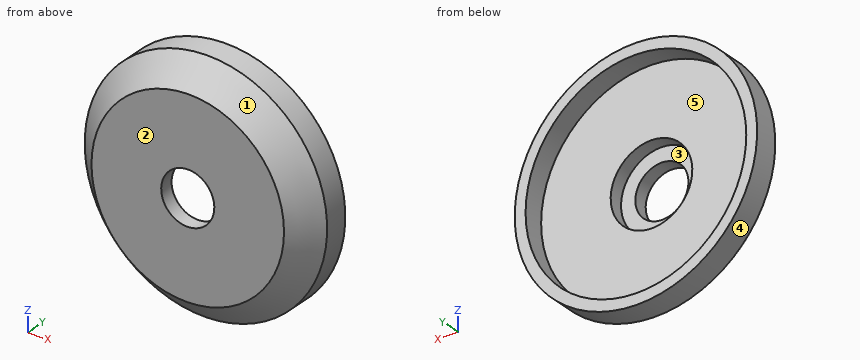
```python
from build123d import *

# Parameters (mm, degrees)
SKETCH1_R           = 34
BOSS_EXTRUDE1_DEPTH = 14
SKETCH2_R           = 30.95
CUT_EXTRUDE1_DEPTH  = 6
SKETCH3_R           = 11.45
CUT_EXTRUDE2_DEPTH  = 4
SKETCH4_R           = 7.45
CUT_EXTRUDE3_DEPTH  = 4
CHAMFER1_SIZE       = 7


with BuildPart() as part:
    # Sketch1 → Boss-Extrude1 (new body)
    with BuildSketch(Plane(origin=(0, 0, 0), x_dir=(1, 0, 0), z_dir=(0, 1, 0))):
        with Locations(Location((0, 0, 0), (0, 0, 270))):
            Circle(SKETCH1_R)
    extrude(amount=BOSS_EXTRUDE1_DEPTH)

    # Sketch2 → Cut-Extrude1 (cut)
    with BuildSketch(Plane(origin=(0, 14, 0), x_dir=(1, 0, 0), z_dir=(0, 1, 0))):
        with Locations(Location((0, 0, 0), (0, 0, 270))):
            Circle(SKETCH2_R)
    extrude(amount=-CUT_EXTRUDE1_DEPTH, mode=Mode.SUBTRACT)

    # Sketch3 → Cut-Extrude2 (cut)
    with BuildSketch(Plane(origin=(0, 8, 0), x_dir=(1, 0, 0), z_dir=(0, 1, 0))):
        with Locations(Location((0, 0, 0), (0, 0, 270))):
            Circle(SKETCH3_R)
    extrude(amount=-CUT_EXTRUDE2_DEPTH, mode=Mode.SUBTRACT)

    # Sketch4 → Cut-Extrude3 (cut)
    with BuildSketch(Plane(origin=(0, 4, 0), x_dir=(1, 0, 0), z_dir=(0, 1, 0))):
        with Locations(Location((0, 0, 0), (0, 0, 270))):
            Circle(SKETCH4_R)
    extrude(amount=-CUT_EXTRUDE3_DEPTH, mode=Mode.SUBTRACT)

    # Chamfer1
    chamfer1_edges = [part.edges().sort_by_distance(p)[0] for p in [
        (0, 0, -34),
    ]]
    chamfer(chamfer1_edges, length=CHAMFER1_SIZE)


solid = part.part
```
Part model, mm, in its own coordinate system. Face numbers are marked on the shaded views. A direction names the side the tool comes from. Round coordinates to 2 decimals unless told otherwise and drop trailing zeros. Order: outer loops, then holes, each group sorted by start corner. A loop starts at its lowest first (then second) coordinate and runs counter-clockwise, first axis right, second up. Notation, with made-up numbers: M -11.75,43 L 42.25,43 A22 ccw 42.25,68 Z; hole C 16,-11 d4. An arc over 180 degrees is marked long. Put each result on its own line as item: value. Start each with the question number.
1. Drill centre lines: probe 1 along X at (y, z) = (9.4, 0); probe 2 along X at (y, z) = (7.25, 0); probe 3 along Y at (x, z) = (-18, -18). Where is each one in solid material? Low to high. Write a range as [from, to].
2. Two-plate mould, pull along Z, no slides. Class the marked faces 1, 2 and 3: +Z half, -Z half, draft (parallel to the pull), parting line (faces both ways), or undercut.
3. Drop flat-ended pins along their axis: pin 1 (18.5 mm diameter, centred on x = -2.5, z = 5, fed in from +Y); pin 2 (5 mm diameter, centred on x = -17.5, y = 8.5, fed in from -Z); pin 3 (1 mm diameter, centred on y = 4, z = 11, fed in from -X). Give the stop position or say it passes through.
4. Slice it at B-B on z = 0. List the corners of the cut face in (x, y).
5. Tool access for the marked faces 4 and 5: list every direction of +Z, -Z, +X, -X, +Y, -Y with a clear straight run to the whole face (end or side of a thin tool).
6. Slice it at D-D on y = 2.5. List the corners of the cut face in (x, z), then the cut area to 3 significant figures.
7. Slice it at C-C on y = 10. List the corners of the cut face in (x, z).
8. Slice it at A-A on x = 0. List the corners of the cut face in (y, z).
Findings:
1. probe 1: [-34, -30.95], [30.95, 34]
1. probe 2: [-34, -11.45], [11.45, 34]
1. probe 3: [0, 8]
2. face 1: parting line
2. face 2: draft
2. face 3: undercut
3. pin 1: y = 8
3. pin 2: z = -30.51
3. pin 3: x = -29.55
4. outline: M -34,7 L -27,0 L -7.45,0 L -7.45,4 L -11.45,4 L -11.45,8 L -30.95,8 L -30.95,14 L -34,14 Z; M 7.45,0 L 27,0 L 34,7 L 34,14 L 30.95,14 L 30.95,8 L 11.45,8 L 11.45,4 L 7.45,4 Z
5. face 4: +Y, -Y
5. face 5: +Y
6. outline: C 0,0 d59; hole C 0,0 d14.9
6. area: 2,560 mm2
7. outline: C 0,0 d68; hole C 0,0 d61.9
8. outline: M 0,-27 L 7,-34 L 14,-34 L 14,-30.95 L 8,-30.95 L 8,-11.45 L 4,-11.45 L 4,-7.45 L 0,-7.45 Z; M 0,7.45 L 4,7.45 L 4,11.45 L 8,11.45 L 8,30.95 L 14,30.95 L 14,34 L 7,34 L 0,27 Z
